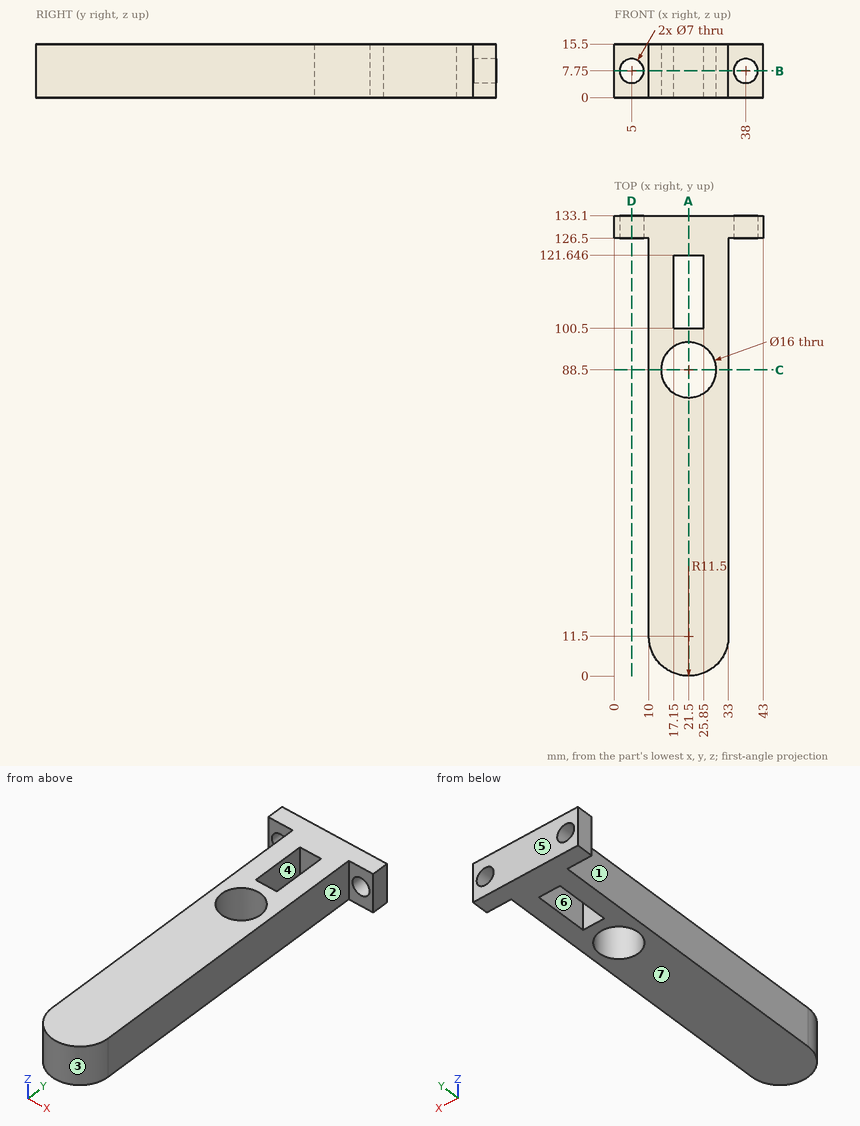
Verification items for this drawing (mm, ordinates from the low corner). A direction names the side the tool comes from. Round coordinates to 2 decimals unless told otherwise and drop trailing zeros. Loops run counter-clockwise (first coordinate to the right, second up) from the corner with the lowest first, then second, coordinate; pieces in that order, holes last. Notation, with made-up numbers: (22.25, 47.5) -> (37.25, 47.5) arc R27 cw to (37.25, 83.5) -> close; hole circle Ø7 at (70.25, 64). An arc over 180 degrees is marked (long way). Write item = value, one per line. Start each with the question number.
1) Sectioned sample at C-C, the plane y = 88.5. Record the cut outline in (x, z).
2) Set-up check for the marked faces 1, 2 and 3: record each of +Z, -Z, +X, -X, +Y, -Y from which the full face is reachable in a straight line by a thin tool's end or side.
3) Sectioned sample at D-D, the plane x = 5. Record the cut outline in (y, z).
4) Sectioned sample at B-B, the plane z = 7.75. Record the cut outline in (x, y).
5) Gauge pin test, flat ends, axial feed: pin 1 Ø8 at (y, z) = (68.5, 11.5) entering from -X; pin 2 Ø5 at (x, z) = (37, 7.5) entering from -Y; pin 3 Ø5 at (x, z) = (13, 9.5) entering from -Y. Record the tip position at first contact, or that the pin passes through.
6) Thickness scan on probe 1 along Y at (x, z) = (21.5, 6); probe 2 along X at (y, z) = (130, 7.75); probe 3 along Y at (x, z) = (20, 4). Record the ranges inside material, lowest first.
7) Sectioned sample at A-A, the plane x = 21.5. Record the cut outline in (y, z).
8) Release check for a two-part mould opening along Y. For the marked faces 4, 5, 6 and 7 record: released by +Y, released by -Y, zero draft, split by the parting line, or undercut.
Results are:
q1.outline = (10, 0) -> (13.5, 0) -> (13.5, 15.5) -> (10, 15.5) -> close; (29.5, 0) -> (33, 0) -> (33, 15.5) -> (29.5, 15.5) -> close
q2.face_1 = +Z, -Z, -X, -Y
q2.face_2 = +Z, -Z, +X, -Y
q2.face_3 = +Z, -Z, -Y
q3.outline = (126.5, 0) -> (133.1, 0) -> (133.1, 4.25) -> (126.5, 4.25) -> close; (126.5, 11.25) -> (133.1, 11.25) -> (133.1, 15.5) -> (126.5, 15.5) -> close
q4.outline = (0, 126.5) -> (1.5, 126.5) -> (1.5, 133.1) -> (0, 133.1) -> close; (8.5, 126.5) -> (10, 126.5) -> (10, 11.5) arc R11.5 ccw to (33, 11.5) -> (33, 126.5) -> (34.5, 126.5) -> (34.5, 133.1) -> (8.5, 133.1) -> close; (41.5, 126.5) -> (43, 126.5) -> (43, 133.1) -> (41.5, 133.1) -> close; hole circle Ø16 at (21.5, 88.5); hole (17.15, 100.5) -> (25.85, 100.5) -> (25.85, 121.65) -> (17.15, 121.65) -> close
q5.pin_1 = 10
q5.pin_2 = 126.5
q5.pin_3 = 1.69
q6.probe_1 = 0 to 80.5, 96.5 to 100.5, 121.65 to 133.1
q6.probe_2 = 0 to 1.5, 8.5 to 34.5, 41.5 to 43
q6.probe_3 = 0.1 to 80.64, 96.36 to 100.5, 121.65 to 133.1
q7.outline = (0, 0) -> (80.5, 0) -> (80.5, 15.5) -> (0, 15.5) -> close; (96.5, 0) -> (100.5, 0) -> (100.5, 15.5) -> (96.5, 15.5) -> close; (121.65, 0) -> (133.1, 0) -> (133.1, 15.5) -> (121.65, 15.5) -> close
q8.face_4 = undercut
q8.face_5 = released by +Y
q8.face_6 = undercut
q8.face_7 = zero draft
